The drawing under review shows one solid part. Ordinate dimensions are in mm from its lowest x, y, z. Give positions to 0.01 mm unless a question says otherwise; leave off trailing zeros. Order: outer loops, then holes, each group sorted by start corner. A loop starts at its lowest first (then second) coordinate and runs counter-clockwise, first axis right, second up. Notation, with made-up numbers: (35, 76.25) -> (92, 76.25) arc R20 ccw to (92, 94.25) -> close; hole circle Ø3 at (66.25, 6). An arc over 180 degrees is marked (long way). One line per item, written item: value. Start each with the question number.
1) Wall thickness on line 1 along Z through (x, y) = (1.05, 4.5); line 2 along Z through (x, y) = (1.3, 2.75); line 3 along Y through (x, z) = (1.25, 15.75): over which ranges is each line inside the solid? List them lowest first. Write a range as from..to.
2) Consider section A-A (z = 15.25). State the section outline as (x, y) points.
3) Consider section C-C (x = 0.8). State how many separate pieces and enclosed holes the cut face has, plus the area to 3 significant figures.
4) The part is to be moulded in two halves that separate along Y. For the marked faces 1, 2, 3 and 4, say which applies: released by +Y, released by -Y, zero draft, split by the parting line, or undercut.
5) Consider section B-B (y = 4.5). State the section outline as (x, z) points.
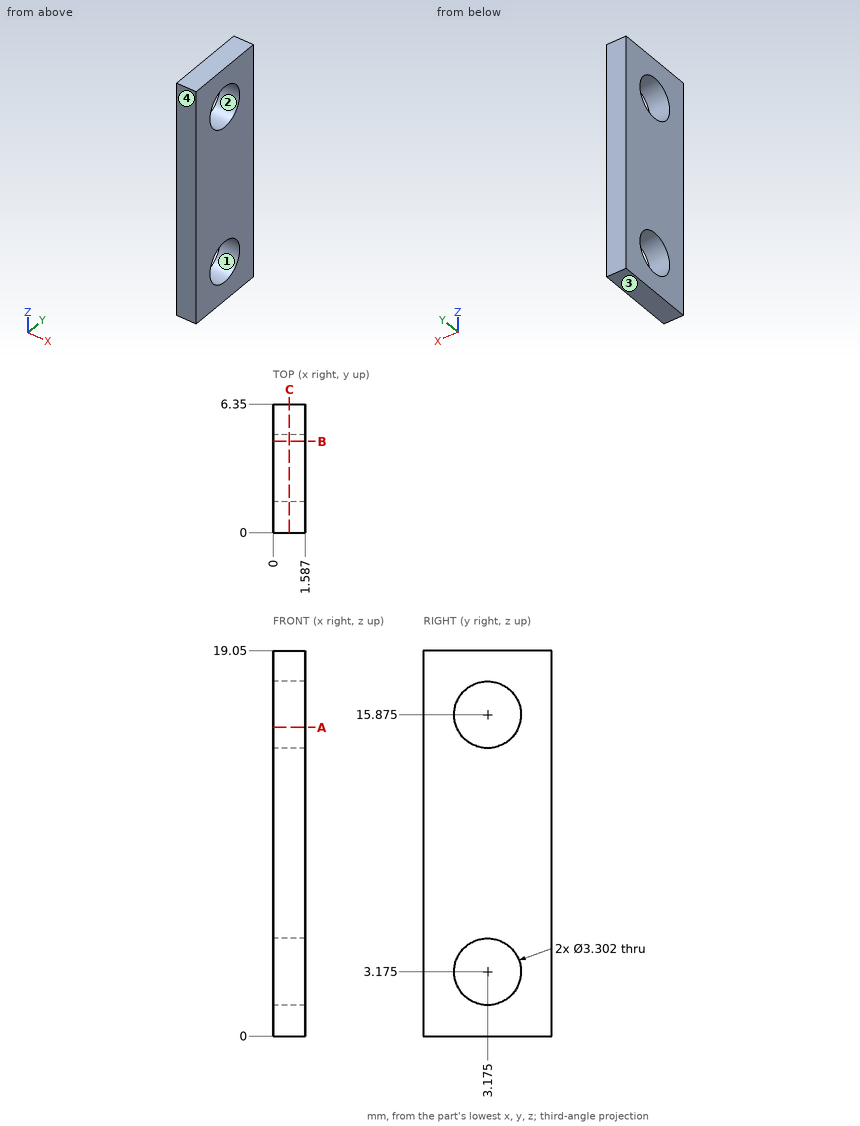
Checked values:
1. line 1: z = 0..2.19, 4.16..14.89, 16.86..19.05
1. line 2: z = 0..1.58, 4.77..14.28, 17.47..19.05
1. line 3: y = 0..1.53, 4.82..6.35
2. outline: (0, 0) -> (1.59, 0) -> (1.59, 1.65) -> (0, 1.65) -> close; (0, 4.7) -> (1.59, 4.7) -> (1.59, 6.35) -> (0, 6.35) -> close
3. separate pieces: 1
3. enclosed holes: 2
3. area: 104 mm^2
4. face 1: undercut
4. face 2: undercut
4. face 3: zero draft
4. face 4: released by -Y
5. outline: (0, 0) -> (1.59, 0) -> (1.59, 2.19) -> (0, 2.19) -> close; (0, 4.16) -> (1.59, 4.16) -> (1.59, 14.89) -> (0, 14.89) -> close; (0, 16.86) -> (1.59, 16.86) -> (1.59, 19.05) -> (0, 19.05) -> close
